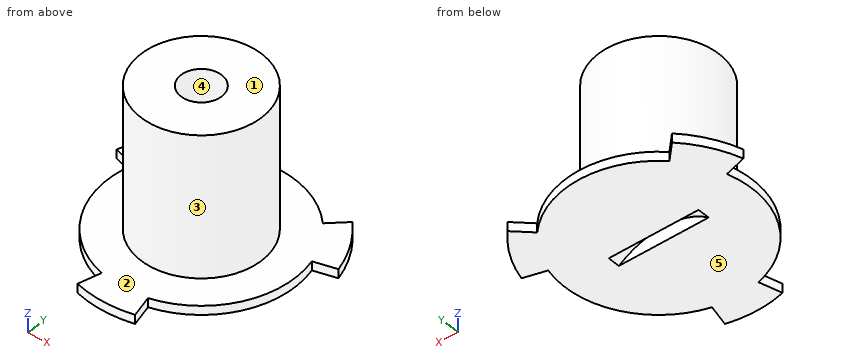
```python
from build123d import *

# Parameters (mm, degrees)
F3_DEPTH = 25.401
F4_R     = 3.429
F5_DEPTH = 19.05
F6_R     = 12.7
F7_DEPTH = 1.016


with BuildPart() as f1:
    # F0 (on Front) → F1 (revolve)
    with BuildSketch(Plane.XZ):
        Polygon((0, 25.4), (0, 0), (19.558, 0), (19.558, 1.524), (10.16, 1.524), (10.16, 25.4), align=None)
    revolve(axis=Axis((0, 0, 10.4228793643), (0, 0, -1)))

    # F2 (on face) → F3 (cut, through all)
    with BuildSketch(Plane(origin=(0, 0, 0), x_dir=(1, 0, 0), z_dir=(0, 0, -1))):
        with BuildLine():
            Line((-3.9429843038, 15.2463890407), (-4.8969321193, 18.9350315505))
            ThreePointArc((-4.8969321193, 18.9350315505), (-16.9377248472, 9.779), (-18.8466844039, -5.2266481593))
            Line((-18.8466844039, -5.2266481593), (-15.1752523771, -4.2084699465))
            ThreePointArc((-15.1752523771, -4.2084699465), (-13.6381680588, 7.874), (-3.9429843038, 15.2463890407))
        make_face()
        with BuildLine():
            Line((4.8969321193, 18.9350315505), (3.9429843038, 15.2463890407))
            ThreePointArc((3.9429843038, 15.2463890407), (13.6381680588, 7.874), (15.1752523771, -4.2084699465))
            Line((15.1752523771, -4.2084699465), (18.8466844039, -5.2266481593))
            ThreePointArc((18.8466844039, -5.2266481593), (19.3793552211, -2.6374144943), (19.558, 0))
            ThreePointArc((19.558, 0), (15.4643066833, 11.9737455629), (4.8969321193, 18.9350315505))
        make_face()
        with BuildLine():
            ThreePointArc((-13.9497522846, -13.7083833912), (0, -19.558), (13.9497522846, -13.7083833912))
            Line((13.9497522846, -13.7083833912), (11.2322680733, -11.0379190942))
            ThreePointArc((11.2322680733, -11.0379190942), (0, -15.748), (-11.2322680733, -11.0379190942))
            Line((-11.2322680733, -11.0379190942), (-13.9497522846, -13.7083833912))
        make_face()
    extrude(amount=-F3_DEPTH, mode=Mode.SUBTRACT)

    # F4 (on face) → F5 (cut)
    with BuildSketch(Plane.XY.offset(25.4)):
        Circle(F4_R)
    extrude(amount=-F5_DEPTH, mode=Mode.SUBTRACT)

    # F6 (on Front) → F7 (cut, symmetric)
    with BuildSketch(Plane.XZ):
        with Locations((0, -10.16)):
            Circle(F6_R)
    extrude(amount=F7_DEPTH, both=True, mode=Mode.SUBTRACT)


solid = f1.part
```
Build history of the part. All positions in model axes, mm. Face numbers are marked on the shaded views. A direction names the side the tool comes from. Give positions to 0.01 mm unless a question says otherwise; leave off trailing zeros. Loops run counter-clockwise (first coordinate to the right, second up) from the corner with the lowest first, then second, coordinate; pieces in that order, holes last.
Item 1: Slice it at D-D, the plane y = 8. List the corners of the cut face in (x, z).
Answers follow:
outline: (-17.85, 0) - (17.85, 0) - (17.85, 1.52) - (6.26, 1.52) - (6.26, 25.4) - (-6.26, 25.4) - (-6.26, 1.52) - (-17.85, 1.52) - close
Item 2: Slice it at A-A, the plane x = 0. List the corners of the cut face in (y, z), and give its area (3 significant figures).
Answers follow:
outline: (-19.56, 0) - (-1.02, 0) - (-1.02, 2.54) - (1.02, 2.54) - (1.02, 0) - (15.75, 0) - (15.75, 1.52) - (10.16, 1.52) - (10.16, 25.4) - (3.43, 25.4) - (3.43, 6.35) - (-3.43, 6.35) - (-3.43, 25.4) - (-10.16, 25.4) - (-10.16, 1.52) - (-19.56, 1.52) - close
area: 403 mm2
Item 3: Slice it at C-C, the plane z = 15.5. List the corners of the cut face in (x, y).
Answers follow:
outline: circle Ø20.32 at (0, 0); hole circle Ø6.86 at (0, 0)
Item 4: Which spindle directions (+Z, -Z, +X, -X, +Y, -Y) get a long thin tool onto all of the face, cutting with end or side? Do the marked faces 1 and 2. Say none if no direction does.
Answers follow:
face 1: +Z, +X, -X, +Y, -Y
face 2: +Z
Item 5: Drill centre lines: line 1 (Y direction, x = 0, z = 20.75); line 2 (Z direction, x = 11.5, y = -8); line 3 (X direction, y = 3, z = 4.5). Where is each one in solid material? Low to high.
Answers follow:
line 1: y = -10.16 to -3.43, 3.43 to 10.16
line 2: z = 0 to 1.52
line 3: x = -9.71 to 9.71
Item 6: Flat gauge pins, fed straight in: pin 1 (3 mm diameter, centred on x = 3, z = 1, fed in from +Y); pin 2 (7.5 mm diameter, centred on x = 0, y = 0, fed in from +Z); pin 3 (6 mm diameter, centred on x = 0, y = 0, fed in from +Z); pin 4 (4 mm diameter, centred on y = 0, z = 8, fed in from +X). Where does each tip first touch, or does it go through?
Answers follow:
pin 1: stops at y = 15.68
pin 2: stops at z = 25.4
pin 3: stops at z = 6.35
pin 4: stops at x = 10.16
Item 7: Slice it at B-B, the plane y = 0. List the corners of the cut face in (x, z), and give its area (3 significant figures).
Answers follow:
outline: (-15.75, 0) - (-7.62, 0) arc R12.7 cw to (7.62, 0) - (15.75, 0) - (15.75, 1.52) - (10.16, 1.52) - (10.16, 25.4) - (3.43, 25.4) - (3.43, 6.35) - (-3.43, 6.35) - (-3.43, 25.4) - (-10.16, 25.4) - (-10.16, 1.52) - (-15.75, 1.52) - close
area: 376 mm2
Item 8: Pull direction X, two halves, no side cores. Call the marked faces 3, 4 and 5: released by +X, released by -X, zero draft, split by the parting line, or undercut.
Answers follow:
face 3: split by the parting line
face 4: undercut
face 5: zero draft
